Autodesk Inventor part; units mm, degrees
ref_plane "YZ Plane" through (0, 0, 0) normal (1, 0, 0) x (0, 1, 0)
ref_plane "XZ Plane" through (0, 0, 0) normal (0, 1, 0) x (-1, 0, 0)
ref_plane "XY Plane" through (0, 0, 0) normal (0, 0, 1) x (1, 0, 0)
sketch "Sketch1" plane through (0, 0, 0) normal (0, 0, 1) x (1, 0, 0)
  arc A0 (-3.2, 0) -> (3.2, 0) centre (0, 0) ccw
  arc A1 (-5.5, 0) -> (5.5, 0) centre (0, 0) ccw
  line L0 (-3.2, 0) -> (-5.5, 0)
  line L1 (-5.5, 0) -> (-5.5, 5.5)
  line L2 (-5.5, 5.5) -> (-3.2, 5.5)
  line L3 (-3.2, 5.5) -> (-3.2, 0)
  line L4 (3.2, 0) -> (5.5, 0)
  line L5 (5.5, 0) -> (5.5, 5.5)
  line L6 (5.5, 5.5) -> (3.2, 5.5)
  line L7 (3.2, 5.5) -> (3.2, 0)
  line L8 (-5.5, 0) -> (-5.5, 5.5)
  line L9 (-5.5, 5.5) -> (-10.5, 5.5)
  line L10 (-10.5, 5.5) -> (-10.5, 0)
  line L11 (-10.5, 0) -> (-5.5, 0)
  line L12 (5.5, 0) -> (5.5, 5.5)
  line L13 (5.5, 5.5) -> (10.5, 5.5)
  line L14 (10.5, 5.5) -> (10.5, 0)
  line L15 (10.5, 0) -> (5.5, 0)
  dimension "d0" = 6.4
  dimension "d1" = 11
  dimension "d2" = 5
  dimension "d3" = 5
extrude "Extr-legs" add sketch "Sketch1" along normal blind 20 contours L11 L10 L9 L1 | L5 L13 L14 L15
extrude "Extr-base" add sketch "Sketch1" against normal blind 2.5
sketch "Sketch2" plane through (0, 0, 20) normal (0, 0, 1) x (1, 0, 0)
  circle A0 centre (0, 0) radius 2.2
  circle A1 centre (0, 0) radius 3.5
  line L0 (5.5, 0) -> (10.5, 0)
  line L1 (-10.5, 0) -> (-5.5, 0)
  line L2 (-10.5, 0) -> (-10.5, 5.5)
  line L3 (-10.5, 5.5) -> (10.5, 5.5)
  line L4 (10.5, 5.5) -> (10.5, 0)
  line L5 (10.5, 0) -> (2.2, 0)
  line L6 (-2.2, 0) -> (-10.5, 0)
  dimension "d8" = 4.4
  dimension "d9" = 7
extrude "Extr-top" add sketch "Sketch2" along normal blind 2.5 contours L5 A1 L6 A0 | A0 L6 A1 L5 | A1 L6 L1 L2 L3 L4 L0 L5
properties part number "cage2table-mount-M4(top)-M6(bottom)"
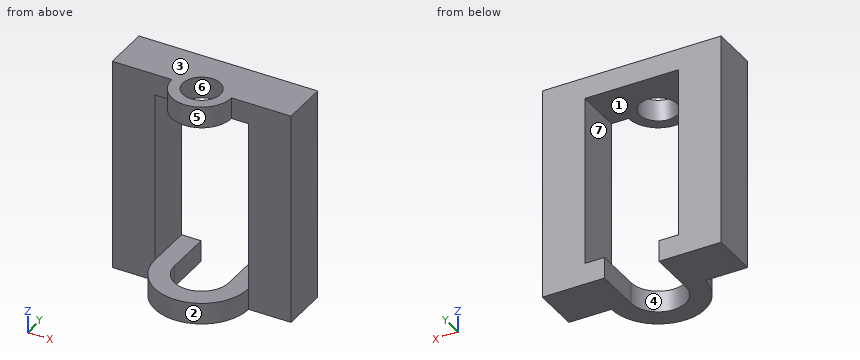
Model file for the job. Use its own axes, mm. Face numbers are marked on the shaded views. A direction names the side the tool comes from. Give positions to 0.01 mm unless a question says otherwise; leave off trailing zeros. Order: outer loops, then holes, each group sorted by start corner. A loop starts at its lowest first (then second) coordinate and runs counter-clockwise, first axis right, second up.
1) Saw through at C-C, the plane y = 1.5. Write the cut outline in (x, z), then the cut area to 3 significant figures.
2) Saw through at D-D, the plane y = -2.5. Write the cut outline in (x, z), then the cut area to 3 significant figures.
3) Pin check, flat tips, straight feed: pin 1 (3.5 mm diameter, centred on x = -6, z = 10, fed in from -Y); pin 2 (3 mm diameter, centred on x = 2, y = -2, fed in from -Z). Stop position of each tip, or through.
4) 3-axis set-ups, long thin cutter, end or side, ignore diameter. For the marked faces 4, 5, 6 and 7: which of +Z, -Z, +X, -X, +Y, -Y reach the whole face in a straight line?
5) Mould opens along X. For the marked faces 1, 2 and 3 say: +X half, -X half, draft (parallel to the pull), parting line (faces both ways), or undercut.
6) Saw through at B-B, the plane z = 14.25. Write the cut outline in (x, y).
7) Saw through at A-A, the plane x = 0. Write the cut outline in (y, z), then the cut area to 4 significant figures.
8) Wall check: probe 1 along X at (y, z) = (3.25, 11.75); probe 2 along Y at (x, z) = (0, 20.95); probe 3 along X at (y, z) = (2.75, -1.5). Give the ranges that are in metal, low to high.
Computed:
1. outline: (-10.5, -2.5) - (-3.2, -2.5) - (-3.2, 0) - (-5.5, 0) - (-5.5, 20) - (-1.61, 20) - (-1.61, 22.5) - (-10.5, 22.5) - close; (1.61, 20) - (5.5, 20) - (5.5, 0) - (3.2, 0) - (3.2, -2.5) - (10.5, -2.5) - (10.5, 22.5) - (1.61, 22.5) - close
1. area: 281 mm2
2. outline: (-4.9, -2.5) - (-2, -2.5) - (-2, 0) - (-4.9, 0) - close; (-2.45, 20) - (2.45, 20) - (2.45, 22.5) - (-2.45, 22.5) - close; (2, -2.5) - (4.9, -2.5) - (4.9, 0) - (2, 0) - close
2. area: 26.8 mm2
3. pin 1: stops at y = 0
3. pin 2: stops at z = -2.5
4. face 4: -Z, +Y
4. face 5: +Z, -Y
4. face 6: +Z, -Z
4. face 7: +Y, -Y
5. face 1: undercut
5. face 2: parting line
5. face 3: draft
6. outline: (-10.5, 0) - (-5.5, 0) - (-5.5, 5.5) - (-10.5, 5.5) - close; (5.5, 0) - (10.5, 0) - (10.5, 5.5) - (5.5, 5.5) - close
7. outline: (-5.5, -2.5) - (-3.2, -2.5) - (-3.2, 0) - (-5.5, 0) - close; (-3.5, 20) - (-2.2, 20) - (-2.2, 22.5) - (-3.5, 22.5) - close; (2.2, 20) - (5.5, 20) - (5.5, 22.5) - (2.2, 22.5) - close
7. area: 17.25 mm2
8. probe 1: x = -10.5 to -5.5, 5.5 to 10.5
8. probe 2: y = -3.5 to -2.2, 2.2 to 5.5
8. probe 3: x = -10.5 to -3.2, 3.2 to 10.5
